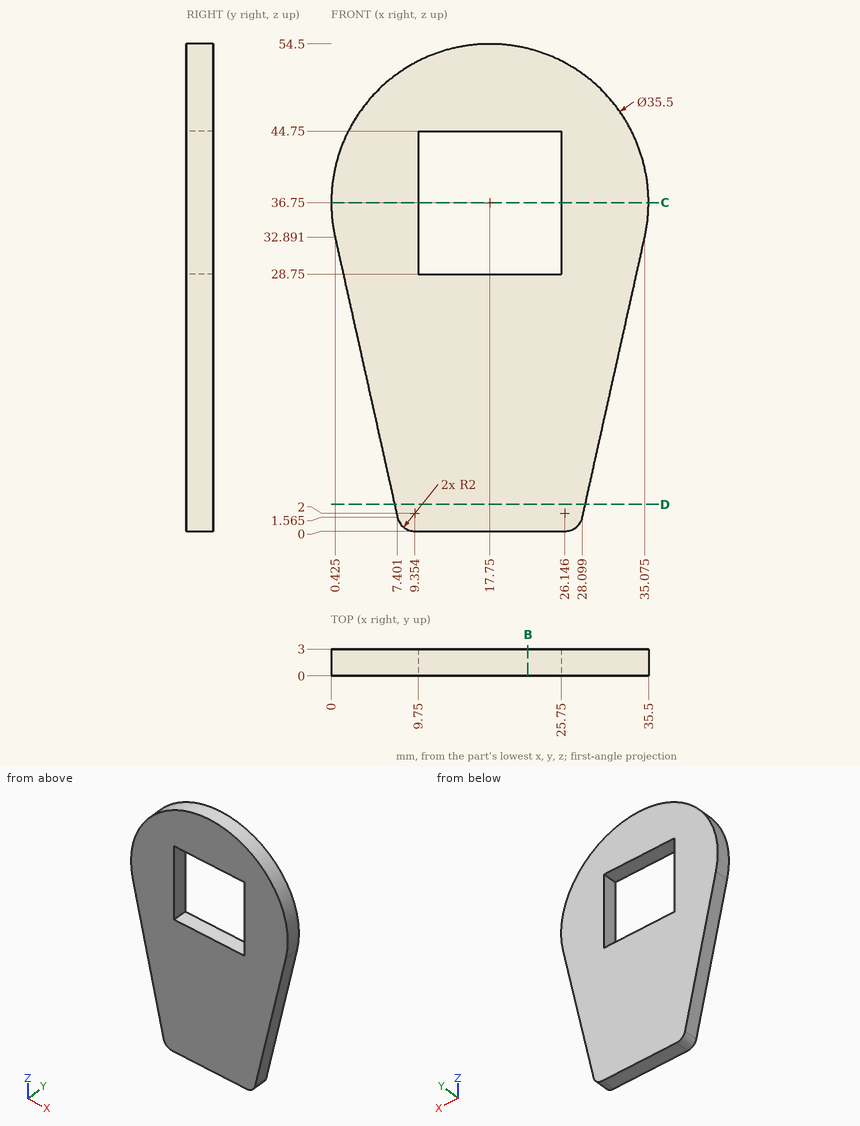
Study the drawing (mm; zero at the part's minimum x, y, z) and answer. Give positions to 0.01 mm unless a question says otherwise; leave off trailing zeros. Write each loop counter-clockwise with the first axis right and the second up, starting at its lowest first coordinate (ties: lowest second). Pieces come first, ordered by that corner, then holes. Notation, with made-up numbers: M 31.5,-6 L 88.5,-6 A17 cw 88.5,6 Z; hole C -24,32.25 d6. An arc over 180 degrees is marked long. Put each result on its own line as item: value. Start each with the question number.
1. The part is cut by section C-C, the plane z = 36.75. Give the vertices of the cut face in (x, y).
2. Consider line 1 along Z through (x, y) = (17.5, 2.1); line 2 along X through (y, z) = (0.35, 37); line 3 along X through (y, z) = (2.5, 40). Determine where each line is inside the solid, lowest interval first.
3. The part is cut by section B-B, the plane x = 22. Give the vertices of the cut face in (y, z).
4. Each of these flat-tipped pins is pushed along its axis until it touches: pin 1 Ø1.5 at (x, y) = (9.5, 2) entering from +Z; pin 2 Ø10 at (x, z) = (18.5, 22.5) entering from -Y; pin 3 Ø0.9 at (x, y) = (19.5, 1) entering from +Z; pin 4 Ø0.9 at (y, z) = (2, 36) entering from -X. Where does it stop, or does it pass through?
5. The part is cut by section D-D, the plane z = 3. Give the vertices of the cut face in (x, y).
Final values:
1. outline: M 0,0 L 9.75,0 L 9.75,3 L 0,3 Z; M 25.75,0 L 35.5,0 L 35.5,3 L 25.75,3 Z
2. line 1: z = 0 to 28.75, 44.75 to 54.5
2. line 2: x = 0 to 9.75, 25.75 to 35.5
2. line 3: x = 0.3 to 9.75, 25.75 to 35.2
3. outline: M 0,0 L 3,0 L 3,28.75 L 0,28.75 Z; M 0,44.75 L 3,44.75 L 3,53.98 L 0,53.98 Z
4. pin 1: stops at z = 52.84
4. pin 2: stops at y = 0
4. pin 3: stops at z = 54.45
4. pin 4: stops at x = 0
5. outline: M 7.08,0 L 28.42,0 L 28.42,3 L 7.08,3 Z
